Work out the finished part from the listing and answer in its coordinate system (mm). Face numbers are marked on the shaded views. A direction names the side the tool comes from. Coordinates: 2 decimals unless noted, no trailing zeros. Order: outer loops, then holes, each group sorted by start corner. A loop starts at its lowest first (then second) coordinate and runs counter-clockwise, first axis right, second up. Notation, with made-up numbers: (-11.5, -4.5) -> (0.5, -4.5) arc R27 ccw to (0.5, 25.5) -> close; hole circle Ø8 at (-9, -30). An arc over 180 degrees is marked (long way). Use one line per item in the form item = value.
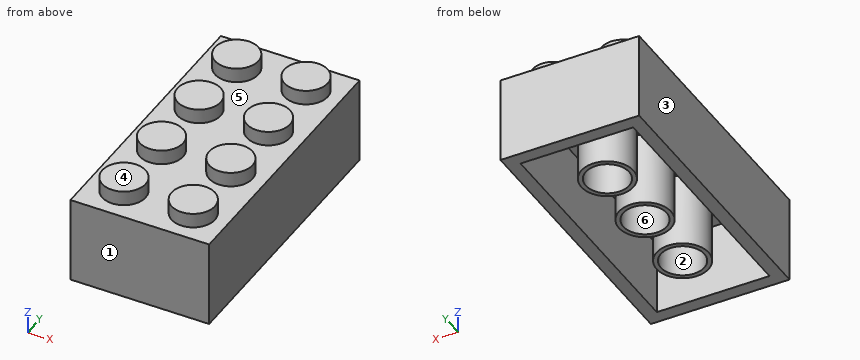
from build123d import *

# Parameters (mm, degrees)
F0_W     = 16
F0_H     = 32
F1_DEPTH = 10
F2_R     = 2.5
F3_DEPTH = 1.7
F4_T     = -1.5
F5_R     = 3
F6_DEPTH = 8.5
F7_T     = -0.5


with BuildPart() as f1:
    # F0 (on Top) → F1 (new body)
    with BuildSketch(Plane.XY):
        with Locations((8, -58.6142044663)):
            Rectangle(F0_W, F0_H)
    extrude(amount=F1_DEPTH)

    # F2 (on face) → F3 (join)
    with BuildSketch(Plane.XY.offset(10)):
        with Locations((4, -46.6142044663)):
            Circle(F2_R)
        with Locations((4, -54.6142044663)):
            Circle(F2_R)
        with Locations((4, -62.6142044663)):
            Circle(F2_R)
        with Locations((4, -70.6142044663)):
            Circle(F2_R)
        with Locations((12, -70.6142044663)):
            Circle(F2_R)
        with Locations((12, -62.6142044663)):
            Circle(F2_R)
        with Locations((12, -54.6142044663)):
            Circle(F2_R)
        with Locations((12, -46.6142044663)):
            Circle(F2_R)
    extrude(amount=F3_DEPTH)

    # F4
    f4_openings = [f1.faces().sort_by_distance(p)[0] for p in [
        (8, -58.614204, 0),
    ]]
    offset(amount=F4_T, openings=f4_openings, kind=Kind.INTERSECTION)

    # F5 (on face) → F6 (join)
    with BuildSketch(Plane(origin=(0, 0, 8.5), x_dir=(1, 0, 0), z_dir=(0, 0, -1))):
        with Locations((8, 66.6142044663)):
            Circle(F5_R)
        with Locations((8, 58.6142044663)):
            Circle(F5_R)
        with Locations((8, 50.6142044663)):
            Circle(F5_R)
    extrude(amount=F6_DEPTH)

    # F7
    f7_openings = [f1.faces().sort_by_distance(p)[0] for p in [
        (8, -66.614204, 0),
        (8, -58.614204, 0),
        (8, -50.614204, 0),
    ]]
    offset(amount=F7_T, openings=f7_openings, kind=Kind.INTERSECTION)


solid = f1.part
(1) Each of these flat-tipped pins is pushed along its axis until it touches: P1, Ø3, axis at x = 12, y = -62.61, coming from the -Z side; P2, Ø6, axis at x = 8, y = -58.61, coming from the +Z side. Where does it stop, or does it pass through?
Data:
P1 = 8.5
P2 = 10
(2) Section A-A on z = 5.5 is taken. Count the separate pieces of the cut face and the enclosed holes in it, plus the area to 3 significant figures.
Data:
separate_pieces = 5
enclosed_holes = 5
area = 116 mm²
(3) The mould has two halves that part along Y. Classify the marked faces 1, 2 and 3: released by +Y, released by -Y, zero draft, split by the parting line, or undercut.
Data:
face_1 = released by -Y
face_2 = undercut
face_3 = zero draft
(4) Straight lines are drawn through the part: line 1 along X through (y, z) = (-45, 5.75); line 2 along Y through (x, z) = (11.75, 1.25); line 3 along Z through (x, y) = (12.5, -44). For each, find the intervals that lie inside material, in ascending order.
Data:
line_1 = 0 to 0.5, 1 to 1.5, 14.5 to 15, 15.5 to 16
line_2 = -74.61 to -74.11, -73.61 to -73.11, -44.11 to -43.61, -43.11 to -42.61
line_3 = 0 to 9, 9.5 to 10
(5) Which of the six approach directions +Z, -Z, +X, -X, +Y, -Y give full straight-line access (tool end or side, diameter ignored) to the marked faces 4, 5 and 6?
Data:
face_4 = +Z, +X, -X, +Y, -Y
face_5 = +Z
face_6 = -Z
(6) Section D-D on y = -66 is taken. Write down the section's boundary in (x, z), plus the area to 3 significant figures.
Data:
outline = (0, 0) -> (1.5, 0) -> (1.5, 8.5) -> (5.06, 8.5) -> (5.06, 0) -> (5.58, 0) -> (5.58, 9) -> (1, 9) -> (1, 0.5) -> (0.5, 0.5) -> (0.5, 9.5) -> (15.5, 9.5) -> (15.5, 0.5) -> (15, 0.5) -> (15, 9) -> (10.42, 9) -> (10.42, 0) -> (10.94, 0) -> (10.94, 8.5) -> (14.5, 8.5) -> (14.5, 0) -> (16, 0) -> (16, 10) -> (0, 10) -> close
area = 39.8 mm²
(7) Section C-C on y = -51 is taken. Write down the section's boundary in (x, z), plus the area to 3 significant figures.
Data:
outline = (0, 0) -> (1.5, 0) -> (1.5, 8.5) -> (5.02, 8.5) -> (5.02, 0) -> (5.53, 0) -> (5.53, 9) -> (1, 9) -> (1, 0.5) -> (0.5, 0.5) -> (0.5, 9.5) -> (15.5, 9.5) -> (15.5, 0.5) -> (15, 0.5) -> (15, 9) -> (10.47, 9) -> (10.47, 0) -> (10.98, 0) -> (10.98, 8.5) -> (14.5, 8.5) -> (14.5, 0) -> (16, 0) -> (16, 10) -> (0, 10) -> close
area = 39.6 mm²
